```python
from build123d import *

# Parameters (mm, degrees)
F0_W      = 137.5
F0_H      = 10
F1_DEPTH  = 9
F3_DEPTH  = 10
F5_DEPTH  = 1.75
F7_DEPTH  = 1.75
F9_DEPTH  = 1.75
F10_R     = 1.5
F11_DEPTH = 134.751
F12_R     = 3.25
F13_DEPTH = 31.6046517502
F15_DEPTH = 134.751
F16_R     = 5.625
F16_R_2   = 3.25
F17_DEPTH = 3


with BuildPart() as f1:
    # F0 (on Top) → F1 (new body)
    with BuildSketch(Plane.XY):
        Rectangle(F0_W, F0_H)
    extrude(amount=F1_DEPTH)

    # F2 (on face) → F3 (join, through all)
    with BuildSketch(Plane(origin=(0, 5, 0), x_dir=(-1, 0, 0), z_dir=(0, 1, 0))):
        with BuildLine():
            Line((-61, -22.6036517502), (-61, -17.1882267114))
            ThreePointArc((-61, -17.1882267114), (-63.7309525503, -16.342729426), (-66, -14.6036517502))
            Line((-66, -14.6036517502), (-66, -22.6036517502))
            Line((-66, -22.6036517502), (-61, -22.6036517502))
        make_face()
        with BuildLine():
            Line((-54, -22.6036517502), (-54, -14.6036517502))
            ThreePointArc((-54, -14.6036517502), (-56.2690474497, -16.342729426), (-59, -17.1882267114))
            Line((-59, -17.1882267114), (-59, -22.6036517502))
            Line((-59, -22.6036517502), (-54, -22.6036517502))
        make_face()
        with BuildLine():
            Line((-1, -22.6036517502), (-1, -17.1882267114))
            ThreePointArc((-1, -17.1882267114), (-3.7309525503, -16.342729426), (-6, -14.6036517502))
            Line((-6, -14.6036517502), (-6, -22.6036517502))
            Line((-6, -22.6036517502), (-1, -22.6036517502))
        make_face()
        with BuildLine():
            ThreePointArc((6, -14.6036517502), (3.7309525503, -16.342729426), (1, -17.1882267114))
            Line((1, -17.1882267114), (1, -22.6036517502))
            Line((1, -22.6036517502), (6, -22.6036517502))
            Line((6, -22.6036517502), (6, -14.6036517502))
        make_face()
        with BuildLine():
            ThreePointArc((59, -17.1882267114), (56.2690474497, -16.342729426), (54, -14.6036517502))
            Line((54, -14.6036517502), (54, -22.6036517502))
            Line((54, -22.6036517502), (59, -22.6036517502))
            Line((59, -22.6036517502), (59, -17.1882267114))
        make_face()
        with BuildLine():
            ThreePointArc((66, -14.6036517502), (63.7309525503, -16.342729426), (61, -17.1882267114))
            Line((61, -17.1882267114), (61, -22.6036517502))
            Line((61, -22.6036517502), (66, -22.6036517502))
            Line((66, -22.6036517502), (66, -14.6036517502))
        make_face()
        with BuildLine():
            ThreePointArc((-1, -13.1269526484), (-2.5387620014, -5.8737982991), (4.125, -9.125))
            ThreePointArc((4.125, -9.125), (3.2512017009, -11.6637620014), (1, -13.1269526484))
            Line((1, -13.1269526484), (1, -17.1882267114))
            ThreePointArc((1, -17.1882267114), (3.7309525503, -16.342729426), (6, -14.6036517502))
            ThreePointArc((6, -14.6036517502), (7.5751443881, -12.0631648184), (8.125, -9.125))
            Line((8.125, -9.125), (8.125, -4))
            Line((8.125, -4), (51.875, -4))
            Line((51.875, -4), (51.875, -9.125))
            ThreePointArc((51.875, -9.125), (52.4248556119, -12.0631648184), (54, -14.6036517502))
            ThreePointArc((54, -14.6036517502), (56.2690474497, -16.342729426), (59, -17.1882267114))
            Line((59, -17.1882267114), (59, -13.1269526484))
            ThreePointArc((59, -13.1269526484), (57.4612379986, -5.8737982991), (64.125, -9.125))
            ThreePointArc((64.125, -9.125), (63.2512017009, -11.6637620014), (61, -13.1269526484))
            Line((61, -13.1269526484), (61, -17.1882267114))
            ThreePointArc((61, -17.1882267114), (63.7309525503, -16.342729426), (66, -14.6036517502))
            ThreePointArc((66, -14.6036517502), (67.5751443881, -12.0631648184), (68.125, -9.125))
            Line((68.125, -9.125), (68.125, -4))
            Line((68.125, -4), (68.75, -4))
            Line((68.75, -4), (68.75, 0))
            Line((68.75, 0), (-68.75, 0))
            Line((-68.75, 0), (-68.75, -4))
            Line((-68.75, -4), (-68.125, -4))
            Line((-68.125, -4), (-68.125, -9.125))
            ThreePointArc((-68.125, -9.125), (-67.5751443881, -12.0631648184), (-66, -14.6036517502))
            ThreePointArc((-66, -14.6036517502), (-63.7309525503, -16.342729426), (-61, -17.1882267114))
            Line((-61, -17.1882267114), (-61, -13.1269526484))
            ThreePointArc((-61, -13.1269526484), (-62.5387620014, -5.8737982991), (-55.875, -9.125))
            ThreePointArc((-55.875, -9.125), (-56.7487982991, -11.6637620014), (-59, -13.1269526484))
            Line((-59, -13.1269526484), (-59, -17.1882267114))
            ThreePointArc((-59, -17.1882267114), (-56.2690474497, -16.342729426), (-54, -14.6036517502))
            ThreePointArc((-54, -14.6036517502), (-52.4248556119, -12.0631648184), (-51.875, -9.125))
            Line((-51.875, -9.125), (-51.875, -4))
            Line((-51.875, -4), (-8.125, -4))
            Line((-8.125, -4), (-8.125, -9.125))
            ThreePointArc((-8.125, -9.125), (-7.5751443881, -12.0631648184), (-6, -14.6036517502))
            ThreePointArc((-6, -14.6036517502), (-3.7309525503, -16.342729426), (-1, -17.1882267114))
            Line((-1, -17.1882267114), (-1, -13.1269526484))
        make_face()
    extrude(amount=-F3_DEPTH)

    # F4 (on face) → F5 (cut)
    with BuildSketch(Plane(origin=(54, 0, 0), x_dir=(0, -1, 0), z_dir=(-1, 0, 0))):
        Polygon((3.7527767497, -17.8536517502), (1.8763883749, -14.6036517502), (-1.8763883749, -14.6036517502), (-3.7527767497, -17.8536517502), (-1.8763883749, -21.1036517502), (1.8763883749, -21.1036517502), align=None)
    extrude(amount=-F5_DEPTH, mode=Mode.SUBTRACT)

    # F6 (on face) → F7 (cut)
    with BuildSketch(Plane.YZ.offset(6)):
        Polygon((3.7527767497, -17.8536517502), (1.8763883749, -14.6036517502), (-1.8763883749, -14.6036517502), (-3.7527767497, -17.8536517502), (-1.8763883749, -21.1036517502), (1.8763883749, -21.1036517502), align=None)
    extrude(amount=-F7_DEPTH, mode=Mode.SUBTRACT)

    # F8 (on face) → F9 (cut)
    with BuildSketch(Plane.YZ.offset(-54)):
        Polygon((1.8763883749, -14.6036517502), (-1.8763883749, -14.6036517502), (-3.7527767497, -17.8536517502), (-1.8763883749, -21.1036517502), (1.8763883749, -21.1036517502), (3.7527767497, -17.8536517502), align=None)
    extrude(amount=-F9_DEPTH, mode=Mode.SUBTRACT)

    # F10 (on face) → F11 (cut, through all)
    with BuildSketch(Plane.YZ.offset(66)):
        with Locations((0.1443375673, -17.8536517502)):
            Circle(F10_R)
    extrude(amount=-F11_DEPTH, mode=Mode.SUBTRACT)

    # F12 (on face) → F13 (cut, through all)
    with BuildSketch(Plane.XY.offset(9)):
        with Locations((36.913, 0)):
            Circle(F12_R)
        with Locations((-36.913, 0)):
            Circle(F12_R)
    extrude(amount=-F13_DEPTH, mode=Mode.SUBTRACT)

    # F14 (on face) → F15 (cut, through all)
    with BuildSketch(Plane.YZ.offset(66)):
        with BuildLine():
            ThreePointArc((-3, -22.6036517502), (-4.4142135624, -22.0178653126), (-5, -20.6036517502))
            Line((-5, -20.6036517502), (-5, -22.6036517502))
            Line((-5, -22.6036517502), (-3, -22.6036517502))
        make_face()
        with BuildLine():
            ThreePointArc((5, -20.6036517502), (4.4142135624, -22.0178653126), (3, -22.6036517502))
            Line((3, -22.6036517502), (5, -22.6036517502))
            Line((5, -22.6036517502), (5, -20.6036517502))
        make_face()
    extrude(amount=-F15_DEPTH, mode=Mode.SUBTRACT)

    # F16 (on face) → F17 (cut)
    with BuildSketch(Plane(origin=(0, 0, -4), x_dir=(1, 0, 0), z_dir=(0, 0, -1))):
        with Locations((-36.913, 0)):
            Circle(F16_R)
        with Locations((-36.913, 0)):
            Circle(F16_R_2, mode=Mode.SUBTRACT)
        with Locations((36.913, 0)):
            Circle(F16_R)
        with Locations((36.913, 0)):
            Circle(F16_R_2, mode=Mode.SUBTRACT)
    extrude(amount=-F17_DEPTH, mode=Mode.SUBTRACT)


solid = f1.part
```
Can you work these out from the model? Positions are in its coordinate system, mm. A direction names the side the tool comes from. Round coordinates to 2 decimals unless told otherwise and drop trailing zeros. Loops run counter-clockwise (first coordinate to the right, second up) from the corner with the lowest first, then second, coordinate; pieces in that order, holes last. Notation, with made-up numbers: (86, 29) -> (138, 29) arc R12 ccw to (138, 43) -> close; hole circle Ø4 at (-30.75, 63.25). An arc over 180 degrees is marked (long way). One line per item, written item: value. Start each with the question number.
1. If I drill on probe 1 along X at (y, z) = (0.5, -20); probe 2 along X at (y, z) = (0, 2); probe 3 along X at (y, z) = (-1, -9) (3 decimals), over which ranges is the centre line in solid material (lowest first)?
2. If we mould it in two halves opening along Z, with no side actions, what happens to faces 1 (the cylindrical face through (-63.46, -0.18, -19.32)), 2 (the flat face through (68.125, 0, -7)), 3 (the flat face through (21, 0, -4))? For each: pulls with the +Z half, pulls with the -Z half, needs draft (parallel to the pull), parting line crosses it, or undercut.
3. If we section it at A-A, the plane x = -35.5: Write out the boundary of the cut face in (y, z).
4. For faces 4 (the flat face through (55.75, -2, -18)), 5 (the cylindrical face through (42.537, 0.086, -2.521)), 6 (the flat face through (-66, 0, -20)), 7 (the flat face through (66, -1, -19.4)), 8 (the flat face through (47, 0, -4)), which set-ups out of +Z, -Z, +X, -X, +Y, -Y let a thin tool reach every point of the face, with its end or its side?
5. For pin 1 (5 mm diameter, centred on x = 37.5, y = 2, fed in from -Z); pin 2 (1.5 mm diameter, centred on y = -2.5, z = -7, fed in from -X) (3 decimals); pin 3 (3 mm diameter, centred on x = -51, y = -4, fed in from -Z), each with a flat end and sliding along its axis, tell me the tip position at first contact or that it passes through.
6. If we section it at B-B, the plane y = 0: Give the number of separate pieces and of enclosed holes in the cut face, then the cut area to 3 significant figures.
Calculated:
1. probe 1: x = -66 to -61, -59 to -55.75, -6 to -1, 1 to 4.25, 55.75 to 59, 61 to 66
1. probe 2: x = -68.75 to -40.16, -33.66 to 33.66, 40.16 to 68.75
1. probe 3: x = -68.125 to -64.123, -55.877 to -51.875, -8.125 to -4.123, 4.123 to 8.125, 51.875 to 55.877, 64.123 to 68.125
2. face 1: undercut
2. face 2: needs draft
2. face 3: pulls with the -Z half
3. outline: (-5, -1) -> (-2.93, -1) -> (-2.93, 9) -> (-5, 9) -> close; (2.93, -1) -> (5, -1) -> (5, 9) -> (2.93, 9) -> close
4. face 4: none
4. face 5: -Z
4. face 6: -Z, -X, +Y, -Y
4. face 7: -Z, +X, +Y, -Y
4. face 8: -Z, +Y, -Y
5. pin 1: stops at z = -1
5. pin 2: stops at x = -68.125
5. pin 3: stops at z = -12.25
6. separate pieces: 9
6. enclosed holes: 0
6. area: 2,050 mm²
